CAD build for the part. Positions are in the model's coordinates, mm. Round coordinates to 2 decimals unless told otherwise and drop trailing zeros. Loops run counter-clockwise (first coordinate to the right, second up) from the corner with the lowest first, then second, coordinate; pieces in that order, holes last.
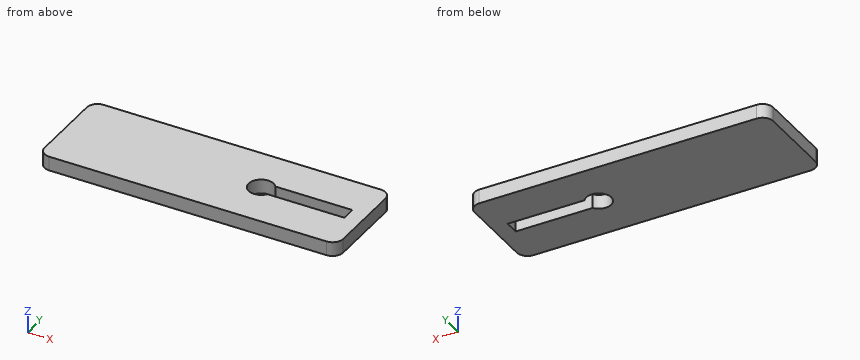
```python
from build123d import *

# Parameters (mm, degrees)
F0_W     = 1066.8
F0_H     = 342.9
F1_DEPTH = 50.8
F2_R     = 38.1
F4_DEPTH = 50.8


with BuildPart() as f1:
    # F0 (on Top) → F1 (new body)
    with BuildSketch(Plane.XY):
        Rectangle(F0_W, F0_H)
    extrude(amount=F1_DEPTH)

    # F2
    f2_edges = [f1.edges().sort_by_distance(p)[0] for p in [
        (-533.4, 171.45, 25.4),
        (-533.4, -171.45, 25.4),
        (533.4, 171.45, 25.4),
        (533.4, -171.45, 25.4),
    ]]
    fillet(f2_edges, radius=F2_R)

    # F3 (on face) → F4 (cut)
    with BuildSketch(Plane.XY.offset(50.8)):
        with BuildLine():
            ThreePointArc((201.577973, -25.4), (207.51019, -13.310834), (209.55, 0))
            ThreePointArc((209.55, 0), (207.51019, 13.310834), (201.577973, 25.4))
            ThreePointArc((201.577973, 25.4), (120.65, 0), (201.577973, -25.4))
        make_face()
        with BuildLine():
            ThreePointArc((201.577973, 25.4), (207.51019, 13.310834), (209.55, 0))
            ThreePointArc((209.55, 0), (207.51019, -13.310834), (201.577973, -25.4))
            Line((201.577973, -25.4), (476.25, -25.4))
            Line((476.25, -25.4), (476.25, 25.4))
            Line((476.25, 25.4), (201.577973, 25.4))
        make_face()
    extrude(amount=-F4_DEPTH, mode=Mode.SUBTRACT)


solid = f1.part
```
Item 1: Cut at B-B, the plane y = 0. Give the cut face in (x, z), plus the area to 3 significant figures.
Answers follow:
outline: (-533.4, 0) - (120.65, 0) - (120.65, 50.8) - (-533.4, 50.8) - close; (476.25, 0) - (533.4, 0) - (533.4, 50.8) - (476.25, 50.8) - close
area: 36,100 mm2
Item 2: Cut at A-A, the plane x = 429. Give the cut face in (y, z), plus the area to 3 significant figures.
Answers follow:
outline: (-171.45, 0) - (-25.4, 0) - (-25.4, 50.8) - (-171.45, 50.8) - close; (25.4, 0) - (171.45, 0) - (171.45, 50.8) - (25.4, 50.8) - close
area: 14,800 mm2
Item 3: Probe line 1 (X direction, y = 0, z = 19); line 2 (Y direction, x = 437.5, z = 39); line 3 (Y direction, x = 165.1, z = 14). List the from-to ranges inside material, lowest first.
Answers follow:
line 1: x = -533.4 to 120.65, 476.25 to 533.4
line 2: y = -171.45 to -25.4, 25.4 to 171.45
line 3: y = -171.45 to -44.45, 44.45 to 171.45
Item 4: Cut at C-C, the plane z = 15. Give the cut face in (x, y).
Answers follow:
outline: (-533.4, -133.35) arc R38.1 ccw to (-495.3, -171.45) - (495.3, -171.45) arc R38.1 ccw to (533.4, -133.35) - (533.4, 133.35) arc R38.1 ccw to (495.3, 171.45) - (-495.3, 171.45) arc R38.1 ccw to (-533.4, 133.35) - close; hole (201.58, -25.4) - (476.25, -25.4) - (476.25, 25.4) - (201.58, 25.4) arc R44.45 ccw (long way) to start
